The figure shows three views and two pictorial views of one solid part (mm, origin at its lowest corner). Answer the questions. A direction names the side the tool comes from. Give positions to 0.01 mm unless a question says otherwise; leave off trailing zeros. Write each loop counter-clockwise with the first axis right and the second up, starting at its lowest first coordinate (ties: lowest second). Pieces come first, ordered by that corner, then holes. Notation, with made-up numbers: (-2.75, -6.5) - (7.25, -6.5) arc R33 cw to (7.25, 25.5) - close; hole circle Ø3 at (80, 34.5). An arc over 180 degrees is marked (long way). Use a Markdown table: item, result. Add a question column.
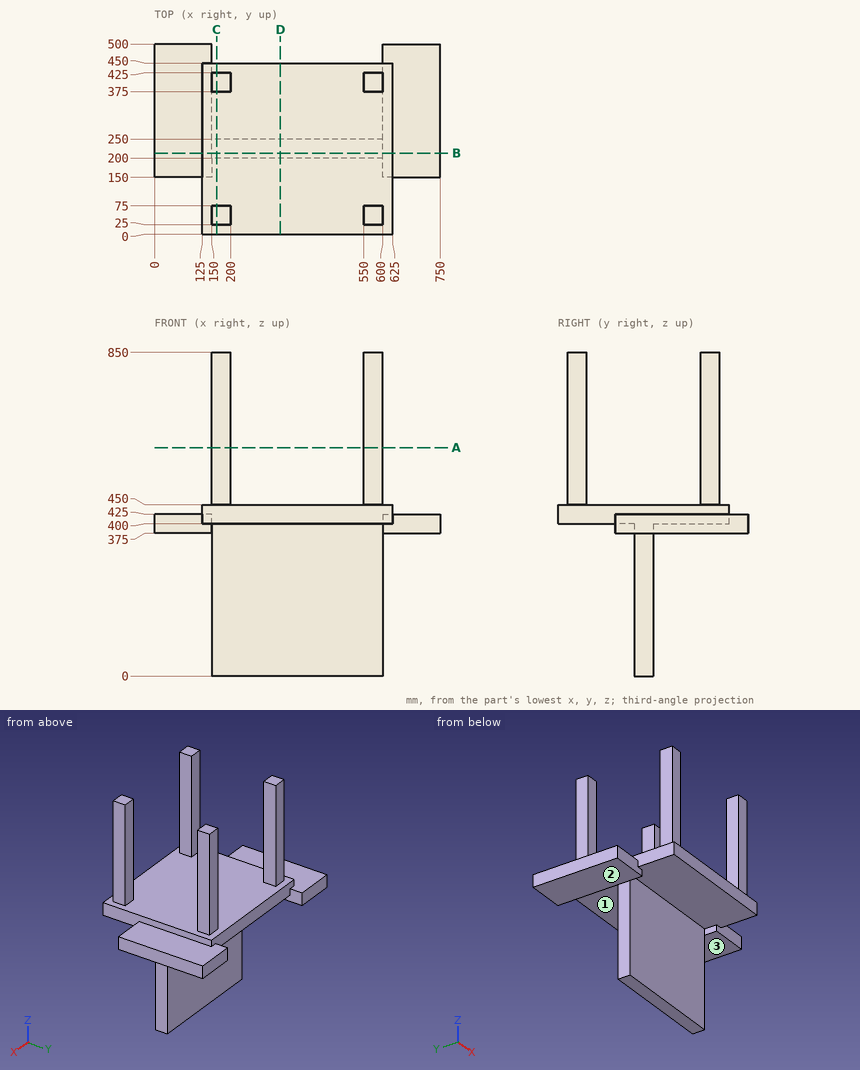
1. Given P1, Ø25, axis at x = 680, z = 402, coming from the -Y side; P2, Ø4, axis at x = 99, y = 309, coming from the +Z side; P3, Ø6, axis at x = 142.5, y = 212.5, coming from the -Z side, each flat-ended and moving along its own axis, determine where each tip first touches the part or whether it passes through.
2. The part is cut by section A-A (z = 599.5). Give the vertices of the cut face in (x, y), and give its area (3 significant figures).
3. The part is cut by section D-D (x = 330.5). Give the vertices of the cut face in (y, z).
4. Which of the six approach directions +Z, -Z, +X, -X, +Y, -Y give full straight-line access (tool end or side, diameter ignored) to the marked faces 1, 2 and 3?
5. The part is cut by section B-B (y = 213.5). Give the vertices of the cut face in (x, z).
6. The part is cut by section C-C (x = 163). Give the vertices of the cut face in (y, z), and give its area (3 significant figures).
7. Consider L1, parallel to X at y = 44, z = 597; L2, parallel to X at y = 311, z = 375.5; L3, parallel to Y at x = 173, z = 193.5. Determine where each line is inside the solid, lowest interval first. Write a range as [from, to].
Check values:
| question | item | result |
|---|---|---|
| 1 | P1 | stops at y = 150 |
| 1 | P2 | stops at z = 425 |
| 1 | P3 | stops at z = 375 |
| 2 | outline | (150, 25) - (200, 25) - (200, 75) - (150, 75) - close; (150, 375) - (200, 375) - (200, 425) - (150, 425) - close; (550, 25) - (600, 25) - (600, 75) - (550, 75) - close; (550, 375) - (600, 375) - (600, 425) - (550, 425) - close |
| 2 | area | 10,000 mm2 |
| 3 | outline | (0, 400) - (200, 400) - (200, 0) - (250, 0) - (250, 400) - (450, 400) - (450, 450) - (0, 450) - close |
| 4 | face 1 | -Z, +Y |
| 4 | face 2 | -Z, -X, +Y, -Y |
| 4 | face 3 | -Z, +X, +Y, -Y |
| 5 | outline | (0, 375) - (150, 375) - (150, 0) - (600, 0) - (600, 375) - (750, 375) - (750, 425) - (625, 425) - (625, 450) - (125, 450) - (125, 425) - (0, 425) - close |
| 6 | outline | (0, 400) - (200, 400) - (200, 0) - (250, 0) - (250, 400) - (450, 400) - (450, 450) - (425, 450) - (425, 850) - (375, 850) - (375, 450) - (75, 450) - (75, 850) - (25, 850) - (25, 450) - (0, 450) - close |
| 6 | area | 82,500 mm2 |
| 7 | L1 | x = [150, 200], [550, 600] |
| 7 | L2 | x = [0, 150], [600, 750] |
| 7 | L3 | y = [200, 250] |
